```python
from build123d import *

# Parameters (mm, degrees)
F0_W     = 76.2
F0_H     = 127
F1_DEPTH = 38.1
F3_DEPTH = 76.201


with BuildPart() as f1:
    # F0 (on Front) → F1 (new body, symmetric)
    with BuildSketch(Plane.XZ):
        Rectangle(F0_W, F0_H)
    extrude(amount=F1_DEPTH, both=True)

    # F2 (on face) → F3 (cut, through all)
    with BuildSketch(Plane.XZ.offset(38.1)):
        Polygon((-38.1, 38.1), (-38.1, -63.5), (-12.7, -63.5), align=None)
    extrude(amount=-F3_DEPTH, mode=Mode.SUBTRACT)


solid = f1.part
```
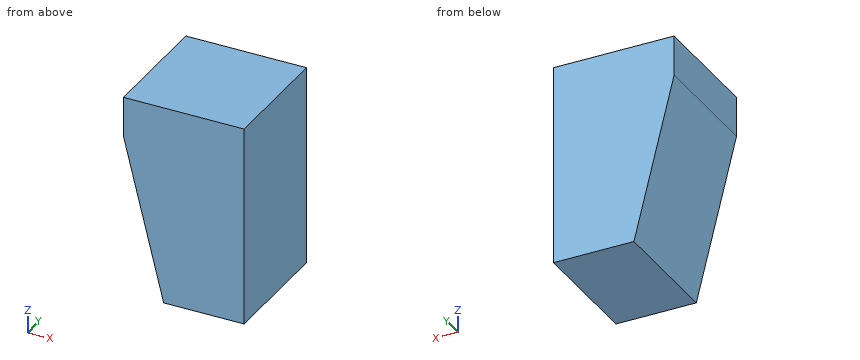
Check sheet for the modelled part. Datum: model origin and axes. Units: mm. Give positions to 0.01 mm unless a question says otherwise; leave off trailing zeros. Order: outer loops, then holes, each group sorted by start corner. A loop starts at its lowest first (then second) coordinate and runs counter-clockwise, first axis right, second up. Notation, with made-up numbers: (24.25, -16.5) -> (66.25, -16.5) arc R20 cw to (66.25, -3.5) -> close; hole circle Ø7 at (58, 65). An arc over 180 degrees is marked (long way). Return JSON: item names as keys, results as strings.
1. Cross-section at A-A, the plane z = 4.5. Record the cut outline in (x, y), plus the area to 3 significant figures.
From the geometry:
{"outline": "(-29.7, -38.1) -> (38.1, -38.1) -> (38.1, 38.1) -> (-29.7, 38.1) -> close", "area": "5,170 mm^2"}
2. Cross-section at C-C, the plane x = -23. Record the cut outline in (y, z), plus the area to 3 significant figures.
From the geometry:
{"outline": "(-38.1, -22.3) -> (38.1, -22.3) -> (38.1, 63.5) -> (-38.1, 63.5) -> close", "area": "6,540 mm^2"}
3. Material ranges on probe 1 along X at (y, z) = (-13, 5.5); probe 2 along X at (y, z) = (9.5, -12) (3 decimals), recorded low to high. Write a range as [from, to].
From the geometry:
{"probe 1": "[-29.95, 38.1]", "probe 2": "[-25.575, 38.1]"}
4. Cross-section at B-B, the plane y = 13.5. Record the cut outline in (x, z).
From the geometry:
{"outline": "(-38.1, 38.1) -> (-12.7, -63.5) -> (38.1, -63.5) -> (38.1, 63.5) -> (-38.1, 63.5) -> close"}
